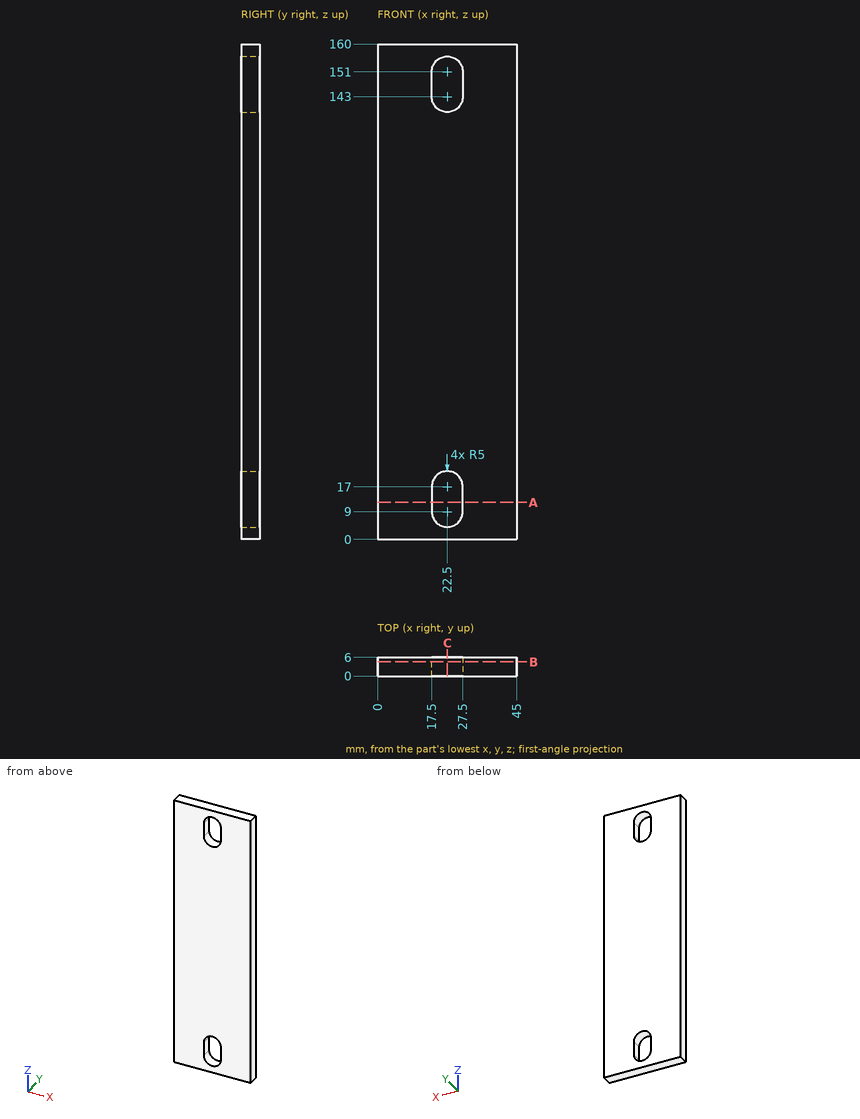
Answer from the drawing. Dimensions are ordinates in mm from the lowest x, y and z of the part. Give positions to 0.01 mm unless a question says otherwise; leave off trailing zeros. Loops run counter-clockwise (first coordinate to the right, second up) from the corner with the lowest first, then second, coordinate; pieces in that order, holes last.
Item 1: The part is cut by section C-C (x = 22.5). Write down the section's boundary in (y, z), and give its area (3 significant figures).
Item 2: This flat-tipped pin is pushed along its axis until it touches: pin 1 Ø1.8 at (y, z) = (2, 145.5) entering from -X. Where does it stop, or does it pass through?
Item 3: Find the intervals of material crossed by line 1 along Z through (x, y) = (22, 3.4); line 2 along Z through (x, y) = (24, 3.45); line 3 along X through (y, z) = (2.85, 149.5), in increasing order.
Item 4: The part is cut by section B-B (y = 4.6). Write down the section's boundary in (x, z), and give its area (3 significant figures).
Item 5: The part is cut by section A-A (z = 12). Write down the section's boundary in (x, y).
Taken from the geometry:
1. outline: (0, 0) - (6, 0) - (6, 4) - (0, 4) - close; (0, 22) - (6, 22) - (6, 138) - (0, 138) - close; (0, 156) - (6, 156) - (6, 160) - (0, 160) - close
1. area: 744 mm2
2. pin 1: stops at x = 0
3. line 1: z = 0 to 4.03, 21.97 to 138.03, 155.97 to 160
3. line 2: z = 0 to 4.23, 21.77 to 138.23, 155.77 to 160
3. line 3: x = 0 to 17.5, 27.5 to 45
4. outline: (0, 0) - (45, 0) - (45, 160) - (0, 160) - close; hole (17.5, 9) arc R5 ccw to (27.5, 9) - (27.5, 17) arc R5 ccw to (17.5, 17) - close; hole (17.5, 143) arc R5 ccw to (27.5, 143) - (27.5, 151) arc R5 ccw to (17.5, 151) - close
4. area: 6,880 mm2
5. outline: (0, 0) - (17.5, 0) - (17.5, 6) - (0, 6) - close; (27.5, 0) - (45, 0) - (45, 6) - (27.5, 6) - close
